Source: CAD feature listing. Evaluate the final solid. Frame: model axes, mm. A direction names the side the tool comes from. Coordinates: 2 decimals unless noted, no trailing zeros. Loops run counter-clockwise (first coordinate to the right, second up) from the corner with the lowest first, then second, coordinate; pieces in that order, holes last.
Item 1: Section query B-B, the plane x = 0. Return the cut outline in (y, z).
Item 2: Pin query (flat end, axial travel): pin 1 Ø1.5 at (x, z) = (15.5, 15) entering from -Y. Return the tip coordinate at first contact, or that it passes through.
Item 3: Section query C-C, the plane x = -13. Return the cut outline in (y, z).
Item 4: Section query A-A, the plane z = 0. Return the cut outline in (x, y), then the cut area to 3 significant figures.
Item 5: Pull-direction query (Z, two-part tool) for faces 1 (the flat face through (20, 5, -11)), 2 (the flat face through (-10, 5, -15)); classes: +Z half, -Z half, draft (parallel to the pull), parting line (faces both ways), or undercut.
Item 6: Line query: probe 1 along X at (y, z) = (5.75, -13); probe 2 along Z at (x, y) = (-16.5, 5.5); probe 3 along X at (y, z) = (3.5, 0). Output: solid intervals per line, ascending.
Item 7: Section query D-D, the plane y = 5. State how many separate pieces and enclosed holes the cut face has, then the cut area to 3 significant figures.
Item 8: Reachability of faces 3 (the flat face through (-4.5, 5, -18)), 4 (the flat face through (10, 5, 15)) from +Z, -Z, +X, -X, +Y, -Y: full face, straight path, thin tool, end or side. Return the list, or none.
```python
from build123d import *

# Parameters (mm, degrees)
SKETCH_1_R      = 3.5
EXTRUDE_1_DEPTH = 10


with BuildPart() as part:
    # 草图1 → 凸台-拉伸1 (new body)
    with BuildSketch(Plane(origin=(0, 0, 0), x_dir=(1, 0, 0), z_dir=(0, 1, 0))):
        with BuildLine():
            Line((11.701656746, 9.664363839), (8.252590681, 5.784164516))
            ThreePointArc((8.252590681, 5.784164516), (8.065278298, 5.475181235), (8, 5.119800678))
            Line((8, 5.119800678), (8, -5.119800678))
            ThreePointArc((8, -5.119800678), (8.065278298, -5.475181235), (8.252590681, -5.784164516))
            Line((8.252590681, -5.784164516), (11.701656746, -9.664363839))
            ThreePointArc((11.701656746, -9.664363839), (12.039410013, -9.912240056), (12.449066064, -10))
            Line((12.449066064, -10), (17.5, -10))
            ThreePointArc((17.5, -10), (17.853553391, -9.853553391), (18, -9.5))
            Line((18, -9.5), (18, -7.5))
            Line((18, -7.5), (15.5, -7.5))
            Line((15.5, -7.5), (15.5, -5.5))
            ThreePointArc((15.5, -5.5), (15.792893219, -4.792893219), (16.5, -4.5))
            Line((16.5, -4.5), (20, -4.5))
            Line((20, -4.5), (20, -17))
            ThreePointArc((20, -17), (19.121320344, -19.121320344), (17, -20))
            Line((17, -20), (4.5, -20))
            Line((4.5, -20), (4.5, -16.5))
            ThreePointArc((4.5, -16.5), (4.792893219, -15.792893219), (5.5, -15.5))
            Line((5.5, -15.5), (7.5, -15.5))
            Line((7.5, -15.5), (7.5, -18))
            Line((7.5, -18), (9.5, -18))
            ThreePointArc((9.5, -18), (9.853553391, -17.853553391), (10, -17.5))
            Line((10, -17.5), (10, -12.449066064))
            ThreePointArc((10, -12.449066064), (9.912240056, -12.039410013), (9.664363839, -11.701656746))
            Line((9.664363839, -11.701656746), (5.784164516, -8.252590681))
            ThreePointArc((5.784164516, -8.252590681), (5.475181235, -8.065278298), (5.119800678, -8))
            Line((5.119800678, -8), (-5.119800678, -8))
            ThreePointArc((-5.119800678, -8), (-5.475181235, -8.065278298), (-5.784164516, -8.252590681))
            Line((-5.784164516, -8.252590681), (-9.664363839, -11.701656746))
            ThreePointArc((-9.664363839, -11.701656746), (-9.912240056, -12.039410013), (-10, -12.449066064))
            Line((-10, -12.449066064), (-10, -17.5))
            ThreePointArc((-10, -17.5), (-9.853553391, -17.853553391), (-9.5, -18))
            Line((-9.5, -18), (-7.5, -18))
            Line((-7.5, -18), (-7.5, -15.5))
            Line((-7.5, -15.5), (-5.5, -15.5))
            ThreePointArc((-5.5, -15.5), (-4.792893219, -15.792893219), (-4.5, -16.5))
            Line((-4.5, -16.5), (-4.5, -20))
            Line((-4.5, -20), (-17, -20))
            ThreePointArc((-17, -20), (-19.121320344, -19.121320344), (-20, -17))
            Line((-20, -17), (-20, -4.5))
            Line((-20, -4.5), (-16.5, -4.5))
            ThreePointArc((-16.5, -4.5), (-15.792893219, -4.792893219), (-15.5, -5.5))
            Line((-15.5, -5.5), (-15.5, -7.5))
            Line((-15.5, -7.5), (-18, -7.5))
            Line((-18, -7.5), (-18, -9.5))
            ThreePointArc((-18, -9.5), (-17.853553391, -9.853553391), (-17.5, -10))
            Line((-17.5, -10), (-12.449066064, -10))
            ThreePointArc((-12.449066064, -10), (-12.039410013, -9.912240056), (-11.701656746, -9.664363839))
            Line((-11.701656746, -9.664363839), (-8.252590681, -5.784164516))
            ThreePointArc((-8.252590681, -5.784164516), (-8.065278298, -5.475181235), (-8, -5.119800678))
            Line((-8, -5.119800678), (-8, 5.119800678))
            ThreePointArc((-8, 5.119800678), (-8.065278298, 5.475181235), (-8.252590681, 5.784164516))
            Line((-8.252590681, 5.784164516), (-11.701656746, 9.664363839))
            ThreePointArc((-11.701656746, 9.664363839), (-12.039410013, 9.912240056), (-12.449066064, 10))
            Line((-12.449066064, 10), (-17.5, 10))
            ThreePointArc((-17.5, 10), (-17.853553391, 9.853553391), (-18, 9.5))
            Line((-18, 9.5), (-18, 7.5))
            Line((-18, 7.5), (-15.5, 7.5))
            Line((-15.5, 7.5), (-15.5, 5.5))
            ThreePointArc((-15.5, 5.5), (-15.792893219, 4.792893219), (-16.5, 4.5))
            Line((-16.5, 4.5), (-20, 4.5))
            Line((-20, 4.5), (-20, 17))
            ThreePointArc((-20, 17), (-19.121320344, 19.121320344), (-17, 20))
            Line((-17, 20), (-4.5, 20))
            Line((-4.5, 20), (-4.5, 16.5))
            ThreePointArc((-4.5, 16.5), (-4.792893219, 15.792893219), (-5.5, 15.5))
            Line((-5.5, 15.5), (-7.5, 15.5))
            Line((-7.5, 15.5), (-7.5, 18))
            Line((-7.5, 18), (-9.5, 18))
            ThreePointArc((-9.5, 18), (-9.853553391, 17.853553391), (-10, 17.5))
            Line((-10, 17.5), (-10, 12.449066064))
            ThreePointArc((-10, 12.449066064), (-9.912240056, 12.039410013), (-9.664363839, 11.701656746))
            Line((-9.664363839, 11.701656746), (-5.784164516, 8.252590681))
            ThreePointArc((-5.784164516, 8.252590681), (-5.475181235, 8.065278298), (-5.119800678, 8))
            Line((-5.119800678, 8), (5.119800678, 8))
            ThreePointArc((5.119800678, 8), (5.475181235, 8.065278298), (5.784164516, 8.252590681))
            Line((5.784164516, 8.252590681), (9.664363839, 11.701656746))
            ThreePointArc((9.664363839, 11.701656746), (9.912240056, 12.039410013), (10, 12.449066064))
            Line((10, 12.449066064), (10, 17.5))
            ThreePointArc((10, 17.5), (9.853553391, 17.853553391), (9.5, 18))
            Line((9.5, 18), (7.5, 18))
            Line((7.5, 18), (7.5, 15.5))
            Line((7.5, 15.5), (5.5, 15.5))
            ThreePointArc((5.5, 15.5), (4.792893219, 15.792893219), (4.5, 16.5))
            Line((4.5, 16.5), (4.5, 20))
            Line((4.5, 20), (17, 20))
            ThreePointArc((17, 20), (19.121320344, 19.121320344), (20, 17))
            Line((20, 17), (20, 4.5))
            Line((20, 4.5), (16.5, 4.5))
            ThreePointArc((16.5, 4.5), (15.792893219, 4.792893219), (15.5, 5.5))
            Line((15.5, 5.5), (15.5, 7.5))
            Line((15.5, 7.5), (18, 7.5))
            Line((18, 7.5), (18, 9.5))
            ThreePointArc((18, 9.5), (17.853553391, 9.853553391), (17.5, 10))
            Line((17.5, 10), (12.449066064, 10))
            ThreePointArc((12.449066064, 10), (12.039410013, 9.912240056), (11.701656746, 9.664363839))
        make_face()
        with Locations(Location((0, 0, 0), (0, 0, 270))):
            Circle(SKETCH_1_R, mode=Mode.SUBTRACT)
        with BuildLine():
            Line((18, -12), (11.701656746, -12))
            Line((11.701656746, -12), (11.701656746, -18))
            Line((11.701656746, -18), (16, -18))
            ThreePointArc((16, -18), (17.414213562, -17.414213562), (18, -16))
            Line((18, -16), (18, -12))
        make_face(mode=Mode.SUBTRACT)
        with BuildLine():
            Line((12, 18), (12, 11.701656746))
            Line((12, 11.701656746), (18, 11.701656746))
            Line((18, 11.701656746), (18, 16))
            ThreePointArc((18, 16), (17.414213562, 17.414213562), (16, 18))
            Line((16, 18), (12, 18))
        make_face(mode=Mode.SUBTRACT)
        with BuildLine():
            Line((-12, -18), (-12, -11.701656746))
            Line((-12, -11.701656746), (-18, -11.701656746))
            Line((-18, -11.701656746), (-18, -16))
            ThreePointArc((-18, -16), (-17.414213562, -17.414213562), (-16, -18))
            Line((-16, -18), (-12, -18))
        make_face(mode=Mode.SUBTRACT)
        with BuildLine():
            Line((-18, 12), (-11.701656746, 12))
            Line((-11.701656746, 12), (-11.701656746, 18))
            Line((-11.701656746, 18), (-16, 18))
            ThreePointArc((-16, 18), (-17.414213562, 17.414213562), (-18, 16))
            Line((-18, 16), (-18, 12))
        make_face(mode=Mode.SUBTRACT)
    extrude(amount=EXTRUDE_1_DEPTH)


solid = part.part
```
Verdict:
1. outline: (0, -8) - (10, -8) - (10, -3.5) - (0, -3.5) - close; (0, 3.5) - (10, 3.5) - (10, 8) - (0, 8) - close
2. pin 1: passes through
3. outline: (0, -20) - (10, -20) - (10, -18) - (0, -18) - close; (0, -12) - (10, -12) - (10, -10) - (0, -10) - close; (0, 10) - (10, 10) - (10, 11.7) - (0, 11.7) - close; (0, 18) - (10, 18) - (10, 20) - (0, 20) - close
4. outline: (-8, 0) - (-3.5, 0) - (-3.5, 10) - (-8, 10) - close; (3.5, 0) - (8, 0) - (8, 10) - (3.5, 10) - close
4. area: 90.0 mm2
5. face 1: draft
5. face 2: undercut
6. probe 1: x = -20 to -18, -11.7 to -10, 10 to 12, 18 to 20
6. probe 2: z = -20 to -17.94, -12 to -10, -7.5 to -4.5, 4.5 to 7.5, 10 to 11.7, 17.94 to 20
6. probe 3: x = -8 to -3.5, 3.5 to 8
7. separate pieces: 1
7. enclosed holes: 5
7. area: 665 mm2
8. face 3: -Z, +Y, -Y
8. face 4: +Y, -Y
